```python
from build123d import *

# Parameters (mm, degrees)
ARMA_W_DEPTH             = 17.5
FILLET_1_R               = 16
FILLET_2_R               = 10
SKETCH_2_R               = 10
CUT_EXTRUDE_1_DEPTH      = 173.351385257
CUT_EXTRUDE_2_DEPTH      = 170.665111322
CUT_EXTRUDE_2_DEPTH_BACK = 170.665111322
ARMA_T_W                 = 31
ARMA_T_H                 = 21
CUT_EXTRUDE_3_DEPTH      = 170.665111322
SKETCH_5_R               = 4
SKETCH_5_R_2             = 3.25
CUT_EXTRUDE_4_DEPTH      = 173.351385257
CUT_EXTRUDE_5_REACH      = 172.898
SKETCH_6_R               = 3
CHAMFER_1_SIZE           = 0.2


with BuildPart() as part:
    # ArmA-L → ArmA-W (new, symmetric)
    with BuildSketch(Plane.XY):
        with BuildLine():
            Line((12.489995997, 10), (70, 10))
            Line((70, 10), (70, 13))
            Line((70, 13), (168, 13))
            Line((168, 13), (168, -10))
            Line((168, -10), (12.489995997, -10))
            ThreePointArc((12.489995997, -10), (-16, 0), (12.489995997, 10))
        make_face()
    extrude(amount=ARMA_W_DEPTH, both=True)

    # ﾌｨﾚｯﾄ1
    fillet_1_edges = [part.edges().sort_by_distance(p)[0] for p in [
        (168, 13, 0),
    ]]
    fillet(fillet_1_edges, radius=FILLET_1_R)

    # ﾌｨﾚｯﾄ2
    # the kernel refuses this fillet: 10 mm, written as the material it adds along each edge
    with BuildSketch(Plane(origin=(12.489995997, -10, -17.5), x_dir=(1, 0, 0), z_dir=(0, 0, 1))) as fillet_2_piece_1:
        with BuildLine():
            CenterArc((4.123251729, -10), FILLET_2_R, 90, 39.715137232)
            Line((-2.266458935, -2.307692308), (-2.394253148, -2.153846154))
            ThreePointArc((-2.394253148, -2.153846154), (-1.217455031, -1.071125515), (-0.15612495, 0.125))
            Line((-0.15612495, 0.125), (0, 0.2))
            Line((0, 0.2), (4.123251729, 0.2))
            Line((4.123251729, 0.2), (4.123251729, 0))
        make_face()
    extrude(amount=35)
    with BuildSketch(Plane(origin=(12.489995997, 10, -17.5), x_dir=(1, 0, 0), z_dir=(0, 0, 1))) as fillet_2_piece_2:
        with BuildLine():
            CenterArc((4.123251729, 10), FILLET_2_R, 230.284862768, 39.715137232)
            Line((-2.266458935, 2.307692308), (-2.394253148, 2.153846154))
            ThreePointArc((-2.394253148, 2.153846154), (-1.217455031, 1.071125515), (-0.15612495, -0.125))
            Line((-0.15612495, -0.125), (0, -0.2))
            Line((0, -0.2), (4.123251729, -0.2))
            Line((4.123251729, -0.2), (4.123251729, 0))
        make_face()
    extrude(amount=35)
    with BuildSketch(Plane(origin=(70, 10, 17.5), x_dir=(0, 1, 0), z_dir=(0, 0, -1))) as fillet_2_piece_3:
        with BuildLine():
            CenterArc((10, -7.141428429), FILLET_2_R, 134.427004001, 45.572995999)
            Line((0, -7.141428429), (-0.2, -7.141428429))
            Line((-0.2, -7.141428429), (-0.2, 0))
            Line((-0.2, 0), (0, 0.2))
            ThreePointArc((0, 0.2), (1.5, 0.2), (2.86, 0.142828569))
            Line((2.86, 0.142828569), (3, 0))
        make_face()
    extrude(amount=35)

    # ｽｹｯﾁ2 → ｶｯﾄ - 押し出し1 (cut, through all)
    with BuildSketch(Plane.XY.offset(17.5)):
        Circle(SKETCH_2_R)
    extrude(amount=-CUT_EXTRUDE_1_DEPTH, mode=Mode.SUBTRACT)

    # ｽｹｯﾁ3 → ｶｯﾄ - 押し出し2 (cut, two sides: drawn at the far end of the back side and taken through both)
    with BuildSketch(Plane(origin=(0, 0, 0), x_dir=(1, 0, 0), z_dir=(0, 1, 0)).offset(-CUT_EXTRUDE_2_DEPTH_BACK)):
        with BuildLine():
            Line((-16, 15.5), (-16, -15.5))
            Line((-16, -15.5), (18.323482202, -15.5))
            ThreePointArc((18.323482202, -15.5), (24, 0), (18.323482202, 15.5))
            Line((18.323482202, 15.5), (-16, 15.5))
        make_face()
    extrude(amount=CUT_EXTRUDE_2_DEPTH + CUT_EXTRUDE_2_DEPTH_BACK, mode=Mode.SUBTRACT)

    # ArmA-t → ｶｯﾄ - 押し出し3 (cut, through all)
    with BuildSketch(Plane(origin=(0, 0, 0), x_dir=(0, 0, -1), z_dir=(1, 0, 0))):
        with Locations((0, 2.5)):
            Rectangle(ARMA_T_W, ARMA_T_H)
    extrude(amount=CUT_EXTRUDE_3_DEPTH, mode=Mode.SUBTRACT)

    # ｽｹｯﾁ5 → ｶｯﾄ - 押し出し4 (cut, through all)
    with BuildSketch(Plane.XY.offset(17.5)):
        with Locations((155, 3)):
            Circle(SKETCH_5_R)
        with Locations((140, 5)):
            Circle(SKETCH_5_R_2)
    extrude(amount=-CUT_EXTRUDE_4_DEPTH, mode=Mode.SUBTRACT)

    # ｽｹｯﾁ6 → ｶｯﾄ - 押し出し5 (cut, up to next)
    with BuildSketch(Plane.XZ.offset(10), mode=Mode.PRIVATE) as cut_extrude_5_sk1:
        with Locations(Location((155, 0, 0), (0, 0, 270))):
            Circle(SKETCH_6_R)
    cut_extrude_5_tool1 = extrude(cut_extrude_5_sk1.sketch, amount=-CUT_EXTRUDE_5_REACH, mode=Mode.PRIVATE) & part.part
    # ｽｹｯﾁ6 → ｶｯﾄ - 押し出し5 (cut, up to next)
    with BuildSketch(Plane.XZ.offset(10), mode=Mode.PRIVATE) as cut_extrude_5_sk2:
        with Locations(Location((41, 0, 0), (0, 0, 270))):
            Circle(SKETCH_6_R)
    cut_extrude_5_tool2 = extrude(cut_extrude_5_sk2.sketch, amount=-CUT_EXTRUDE_5_REACH, mode=Mode.PRIVATE) & part.part
    add(cut_extrude_5_tool1.solids().sort_by_distance((155, -10, 0))[0], mode=Mode.SUBTRACT)
    add(cut_extrude_5_tool2.solids().sort_by_distance((41, -10, 0))[0], mode=Mode.SUBTRACT)

    # 面取り1
    chamfer_1_edges = [part.edges().sort_by_distance(p)[0] for p in [
        (168, -6.5, 17.5),
        (163.313708499, 8.313708499, -15.5),
        (111, 13, -15.5),
        (24, -8, 0),
        (66.731554918, 10.780455543, -15.5),
        (168, -5.5, -15.5),
        (168, -5.5, 15.5),
        (168, -8, 0),
        (168, -10, 0),
        (151, 3, -17.5),
        (151, 3, -15.5),
        (151, 3, 15.5),
        (151, 3, 17.5),
        (136.75, 5, -17.5),
        (136.75, 5, -15.5),
        (136.75, 5, 15.5),
        (136.75, 5, 17.5),
        (155, -8, 3),
        (155, -10, 3),
        (41, -8, 3),
        (41, -10, 3),
        (111, 13, -17.5),
        (111, 13, 17.5),
        (163.313708499, 8.313708499, -17.5),
        (163.313708499, 8.313708499, 17.5),
        (39.735909649, 10, -17.5),
        (39.735909649, 10, 17.5),
        (92.306623863, -10, -17.5),
        (92.306623863, -10, 17.5),
        (-16, 0, -17.5),
        (-16, 0, 17.5),
        (66.731554918, 10.780455543, -17.5),
        (66.731554918, 10.780455543, 17.5),
        (13.216416623, -10.594600569, -17.5),
        (13.216416623, -10.594600569, 17.5),
        (13.216416623, 10.594600569, -17.5),
        (13.216416623, 10.594600569, 17.5),
        (-10, 0, -17.5),
        (-10, 0, 17.5),
        (24, -10, 0),
        (-10, 0, -15.5),
        (17.468364964, -10, -15.5),
        (13.216416623, -10.594600569, -15.5),
        (-16, 0, -15.5),
        (13.216416623, 10.594600569, -15.5),
        (39.735909649, 10, -15.5),
        (-10, 0, 15.5),
        (13.216416623, -10.594600569, 15.5),
        (17.468364964, -10, 15.5),
        (39.735909649, 10, 15.5),
        (13.216416623, 10.594600569, 15.5),
        (-16, 0, 15.5),
        (168, -6.5, -17.5),
        (66.731554918, 10.780455543, 15.5),
        (163.313708499, 8.313708499, 15.5),
        (111, 13, 15.5),
    ]]
    chamfer(chamfer_1_edges, length=CHAMFER_1_SIZE)


solid = part.part
```
The model under review builds one solid part; all positions refer to its coordinate system, in mm. A direction names the side the tool comes from. Round coordinates to 2 decimals unless told otherwise and drop trailing zeros. Order: outer loops, then holes, each group sorted by start corner. A loop starts at its lowest first (then second) coordinate and runs counter-clockwise, first axis right, second up.
Item 1: To check wall thickness, follow probe 1 along Z at (x, y) = (94.5, -5.5); probe 2 along Y at (x, z) = (0, -16); probe 3 along Y at (x, z) = (140, -16.4). State the ranges of each line that lie inside material, in increasing order.
Working result:
probe 1: z = -17.5 to -15.5, 15.5 to 17.5
probe 2: y = -16 to -10, 10 to 16
probe 3: y = -10 to 1.75, 8.25 to 13
Item 2: For pin 1 (0.8 mm diameter, centred on x = 118, z = 16.5, fed in from +Y); pin 2 (7 mm diameter, centred on x = 41, z = 0, fed in from +Y); pin 3 (10.5 mm diameter, centred on x = 112, z = -7, fed in from -Y), all flat-tipped, find the tip position at first contact; note any pin that passes through.
Working result:
pin 1: stops at y = 13
pin 2: stops at y = -8
pin 3: stops at y = -10
Item 3: Add section B-B, the plane x = 82. State the section outline as (y, z) points, and give its area (3 significant figures).
Working result:
outline: (-10, -17.3) - (-9.8, -17.5) - (12.8, -17.5) - (13, -17.3) - (13, -15.7) - (12.8, -15.5) - (-8, -15.5) - (-8, 15.5) - (12.8, 15.5) - (13, 15.7) - (13, 17.3) - (12.8, 17.5) - (-9.8, 17.5) - (-10, 17.3) - close
area: 154 mm2
Item 4: Machinability: for faces 1 (the cylindrical face through (66.78, 10.8, -16.49)), 2 (the flat face through (92, -8, 0)), 3 (the cylindrical face through (157.53, -9.01, -1.61)), which of the approach directions +Z, -Z, +X, -X, +Y, -Y give a long, thin tool a straight path to every point of the face, cutting with its end or side? Answer none if there is none.
Working result:
face 1: +Z, -Z, +Y
face 2: +X, -X, +Y
face 3: +Y, -Y
Item 5: Add section A-A, the plane z = 0. State the section outline as (x, y) points, and give its area (3 significant figures).
Working result:
outline: (24, -9.8) - (24.2, -10) - (37.8, -10) - (38, -9.8) - (38, -8.2) - (37.8, -8) - (24.2, -8) - (24, -8.2) - close; (44, -9.8) - (44.2, -10) - (151.8, -10) - (152, -9.8) - (152, -8.2) - (151.8, -8) - (44.2, -8) - (44, -8.2) - close; (158, -9.8) - (158.2, -10) - (167.8, -10) - (168, -9.8) - (168, -8.2) - (167.8, -8) - (158.2, -8) - (158, -8.2) - close
area: 264 mm2
Item 6: Add section C-C, the plane y = 5. Count the separate pieces of the cut face and the enclosed holes in it, and give its area (3 significant figures).
Working result:
separate pieces: 8
enclosed holes: 0
area: 601 mm2
Item 7: Draft analysis for pull direction Y (two halves, no side actions). For faces 4 (the flat face through (77, 0, 17.5)), 5 (the cylindrical face through (158.815, 4.201, 16.511)), 6 (the cylindrical face through (163.437, 8.189, 16.489)), state which applies: released by +Y, released by -Y, zero draft, split by the parting line, or undercut.
Working result:
face 4: zero draft
face 5: undercut
face 6: released by +Y
